from build123d import *

# Parameters (mm, degrees)
F0_W      = 19.5
F0_H      = 10.5
F1_DEPTH  = 6.4
F2_R      = 1.1728484487
F3_DEPTH  = 25.4
F5_DEPTH  = 25.4
F6_R      = 1.2132701797
F7_DEPTH  = 1.27
F10_DEPTH = 4
F11_R     = 0.254


with BuildPart() as f1:
    # F0 (on Front) → F1 (new body)
    with BuildSketch(Plane.XZ):
        with Locations((9.75, 5.25)):
            Rectangle(F0_W, F0_H)
    extrude(amount=F1_DEPTH)

    # F2 (on face) → F3 (cut)
    with BuildSketch(Plane.XZ.offset(6.4)):
        with Locations((5, 2.9)):
            Circle(F2_R)
        with Locations((14.5, 2.9)):
            Circle(F2_R)
    extrude(amount=-F3_DEPTH, mode=Mode.SUBTRACT)

    # F4 (on face) → F5 (cut)
    with BuildSketch(Plane.XZ.offset(6.4)):
        Polygon((10.16, 10.5), (0, 10.5), (0, 9.6), (7.62, 9.6), align=None)
    extrude(amount=-F5_DEPTH, mode=Mode.SUBTRACT)

    # F6 (on face) → F7 (join)
    with BuildSketch(Plane.XY.offset(10.5)):
        with Locations((12.5, -3.2)):
            Circle(F6_R)
    extrude(amount=F7_DEPTH)

    # F9 (on offset) → F10 (join)
    with BuildSketch(Plane.XZ.offset(5.2)):
        Polygon((17.6, 11.5844129181), (17.6, 10.5), (17.8, 10.5), (17.8, 11.77), (0.0149307994, 13.1014418994), (0, 12.902), align=None)
    extrude(amount=-F10_DEPTH)

    # F11
    f11_edges = [f1.edges().sort_by_distance(p)[0] for p in [
        (17.8, -3.2, 11.77),
        (17.6, -3.2, 11.584413),
    ]]
    fillet(f11_edges, radius=F11_R)


solid = f1.part
Work out the finished part from the listing and answer in its coordinate system (mm). A direction names the side the tool comes from. Coordinates: 2 decimals unless noted, no trailing zeros. Loops run counter-clockwise (first coordinate to the right, second up) from the corner with the lowest first, then second, coordinate; pieces in that order, holes last. Notation, with made-up numbers: (89, -16.5) -> (114, -16.5) arc R18 cw to (114, -1.5) -> close; hole circle Ø8 at (1.5, 9). An arc over 180 degrees is marked (long way). Write each question's results on one line, items separated by ' | '. Start each with the question number.
1) Flat-ended cylindrical pins translate along their axes: P1, Ø1.3, axis at x = 8.5, z = 12, coming from the +Y side; P2, Ø2, axis at x = 6, y = -3, coming from the +Z side; P3, Ø0.8, axis at y = -3.5, z = 11, coming from the +X side. Find the tip coordinate at first contact, or state that the pin passes through.
2) Find section A-A on y = -1.75. Determine the outline of the cut face in (x, z), then the cut area to 3 significant figures.
3) Find section B-B on z = 2.9. Determine the outline of the cut face in (x, y).
4) Find section C-C on x = 12.5. Determine the outline of the cut face in (y, z), then the cut area to 3 significant figures.
5) Consider line 1 along Z through (x, y) = (5, -2.5); line 2 along X through (y, z) = (-3.5, 2.5); line 3 along Z through (x, y) = (5.25, -1.5). Determine where each line is inside the solid, lowest interval first.
6) Find section D-D on x = 14.5. Determine the outline of the cut face in (y, z).
7) For faces 1 (the flat face through (17.6, -3, 11)), 2 (the flat face through (17.8, -3, 11)), 3 (the flat face through (8.872, -3.245, 10.044)), determine the directions among +Z, -Z, +X, -X, +Y, -Y from which every point of the face is accessible in a straight line to the end or side of a thin tool.
8) The mould has two halves that part along X. Classify faces 4 (the flat face through (0, -3, 5)), 5 (the flat face through (4, -3, 9.6)), 6 (the cylindrical face through (11.288, -3.147, 11.126)): pulls with the +X half, pulls with the -X half, needs draft (parallel to the pull), parting line crosses it, or undercut.
Response values:
1) P1: stops at y = -1.2 | P2: stops at z = 12.73 | P3: stops at x = 17.8
2) outline: (0, 0) -> (19.5, 0) -> (19.5, 10.5) -> (17.8, 10.5) -> (17.8, 11.53) arc R0.25 ccw to (17.56, 11.79) -> (0.01, 13.1) -> (0, 12.9) -> (17.36, 11.6) arc R0.25 cw to (17.6, 11.35) -> (17.6, 10.5) -> (10.16, 10.5) -> (7.62, 9.6) -> (0, 9.6) -> close; hole circle Ø2.35 at (5, 2.9); hole circle Ø2.35 at (14.5, 2.9) | area: 192 mm^2
3) outline: (0, -6.4) -> (3.83, -6.4) -> (3.83, 0) -> (0, 0) -> close; (6.17, -6.4) -> (13.33, -6.4) -> (13.33, 0) -> (6.17, 0) -> close; (15.67, -6.4) -> (19.5, -6.4) -> (19.5, 0) -> (15.67, 0) -> close
4) outline: (-6.4, 0) -> (0, 0) -> (0, 10.5) -> (-1.99, 10.5) -> (-1.99, 11.77) -> (-4.41, 11.77) -> (-4.41, 10.5) -> (-6.4, 10.5) -> close; (-5.2, 11.97) -> (-1.2, 11.97) -> (-1.2, 12.17) -> (-5.2, 12.17) -> close | area: 71.1 mm^2
5) line 1: z = 0 to 1.73, 4.07 to 9.6, 12.53 to 12.73 | line 2: x = 0 to 3.9, 6.1 to 13.4, 15.6 to 19.5 | line 3: z = 0 to 1.75, 4.05 to 9.6, 12.51 to 12.71
6) outline: (-6.4, 0) -> (0, 0) -> (0, 1.73) -> (-6.4, 1.73) -> close; (-6.4, 4.07) -> (0, 4.07) -> (0, 10.5) -> (-6.4, 10.5) -> close; (-5.2, 11.82) -> (-1.2, 11.82) -> (-1.2, 12.02) -> (-5.2, 12.02) -> close
7) face 1: +Y, -Y | face 2: +Z, +X, +Y, -Y | face 3: -X, +Y, -Y
8) face 4: pulls with the -X half | face 5: needs draft | face 6: undercut
